Verification items for the finished model (mm, model axes). A direction names the side the tool comes from. Give positions to 0.01 mm unless a question says otherwise; leave off trailing zeros. Order: outer loops, then holes, each group sorted by start corner. A loop starts at its lowest first (then second) coordinate and runs counter-clockwise, first axis right, second up.
Autodesk Inventor part; units mm, degrees
ref_plane "YZ Plane" through (0, 0, 0) normal (1, 0, 0) x (0, 1, 0)
ref_plane "XZ Plane" through (0, 0, 0) normal (0, 1, 0) x (-1, 0, 0)
ref_plane "XY Plane" through (0, 0, 0) normal (0, 0, 1) x (1, 0, 0)
sketch "Sketch1" plane through (0, 0, 0) normal (1, 0, 0) x (0, 1, 0)
  line L0 (0, 0) -> (0, -9.15) construction
  line L1 (0, -9.15) -> (9.0687, -2.8) construction
  line L2 (9.0687, -2.8) -> (9.0687, 0) construction
  line L3 (0, -9.15) -> (0, -29.4542) construction
  line L4 (0, 0) -> (49.8191, 0) construction
  line L5 (9.0687, 0) -> (0, 0)
  line L6 (9.0687, -2.8) -> (25.35, -2.8)
  line L7 (25.35, -2.8) -> (25.35, 0)
  line L8 (25.35, 0) -> (9.0687, 0)
  line L9 (9.0687, -2.8) -> (0, -4.3991)
  line L10 (0, 0) -> (0, -4.3991)
  dimension "d1" = 125
  dimension "d2" = 5.6
  dimension "d3" = 9.15
  dimension "d5" = 9.0687
  dimension "d6" = 25.35
  dimension "d8" = 80
revolve "Revolution1" add sketch "Sketch1" angle 360 about axis through (0, 0, 0) along (0, 1, 0)
sketch "Sketch2" plane through (0, 0, 0) normal (0, -1, 0) x (1, 0, 0)
  line L0 (6.9, -13.1) -> (-16.1, -13.1) construction
  line L1 (-16.1, -13.1) -> (-16.1, 36.9)
  line L2 (-16.1, 36.9) -> (6.9, 36.9)
  line L3 (6.9, 36.9) -> (6.9, -13.1) construction
  circle A0 centre (0, 0) radius 12.5 construction
  circle A1 centre (0, 0) radius 13 construction
  line L4 (6.9, -13.1) -> (6.9, -11.0177) construction
  line L5 (6.9, 36.9) -> (6.9, 11.0177)
  line L6 (0, -13.1) -> (0, -13) construction
  line L7 (3.9, 12.4012) -> (3.9, 33.9)
  line L8 (3.9, 33.9) -> (-13.1, 33.9)
  line L9 (-13.1, 33.9) -> (-13.1, 0)
  arc A2 (6.9, 11.0177) -> (3.9, 12.4012) centre (0, 0) ccw
  arc A3 (-13.1, 0) -> (0, -13.1) centre (0, 0) ccw
  line L10 (0, -13.1) -> (0, -16.1) construction
  line L11 (-13.1, 0) -> (-13, 0) construction
  circle A4 centre (0, 0) radius 2.8
  line L12 (0, 0) -> (-13, 0) construction
  arc A5 (0, -13.1) -> (6.9, -11.0177) centre (0.1762, -1.2107) ccw
  line L13 (-13.1, 0) -> (-16.1, 0) construction
  arc A6 (-16.1, 0) -> (0, -16.1) centre (0, 0) ccw
  line L14 (6.9, -11.0177) -> (6.9, -14.0177)
  arc A7 (0, -16.1) -> (6.9, -14.0177) centre (0, -3.6267) ccw
  dimension "d9" = 25
  dimension "d10" = 0.5
  dimension "d11" = 3
  dimension "d12" = 3
  dimension "d13" = 3
  dimension "d15" = 3
  dimension "d16" = 23
  dimension "d18" = 0.1
  dimension "d19" = 0.1
  dimension "d22" = 3
  dimension "d23" = 11.8906
  dimension "d24" = 50
extrude "Extrusion1" add sketch "Sketch2" against normal up to surface (25.35 mm away) contours L1 L2 L5 A2 L7 L8 L9 A3 A5 L14 A7 A6
sketch "Sketch3" plane through (0, 0, 0) normal (0, -1, 0) x (1, 0, 0)
  line L0 (6.9, 11.0177) -> (6.9, 36.9)
  line L1 (6.9, 36.9) -> (-16.1, 36.9)
  line L2 (-16.1, 36.9) -> (-16.1, 0)
  arc A0 (-16.1, 0) -> (0, -16.1) centre (0, 0) ccw
  arc A1 (0, -16.1) -> (6.9, -14.0177) centre (0, -3.6267) ccw
  line L3 (6.9, -14.0177) -> (6.9, -11.0177)
  arc A2 (0, -13.1) -> (6.9, -11.0177) centre (0.1762, -1.2107) ccw construction
  line L4 (6.9, 11.0177) -> (6.9, -11.0177) construction
  arc A3 (6.9, -10.4177) -> (6.9, 10.4177) centre (-0.0081, 0) ccw construction
  arc A4 (6.9, -10.6569) -> (6.9, 10.6569) centre (-0.0081, 0) ccw
  line L5 (6.9, 0) -> (12.6919, 0) construction
  line L6 (6.9, -10.6569) -> (6.9, -11.0177)
  line L7 (6.9, 11.0177) -> (6.9, 10.6569)
  point P0 (0, 0)
  dimension "d29" = 12.5
  dimension "d30" = 0.2
  dimension "d31" = 0.6
extrude "Extrusion2" add sketch "Sketch3" along normal blind 3
mirror "Mirror1" about plane through (0, 25.35, 0) normal (0, 1, 0) of "Extrusion1", "Extrusion2", "Revolution1"
(1) Go/stop test with flat-tipped pins: pin 1 (21 mm diameter, centred on y = 31.5, z = 29, fed in from +X); pin 2 (1 mm diameter, centred on x = -6, y = 19.5, fed in from -Z). Record where each tip stops, or that it passes through.
Solved:
pin 1: stops at x = 6.9
pin 2: stops at z = -15.13
(2) Section check B-B, the plane y = 26.5. Enter the section's corners in (x, z), then the cut area to 3 significant figures.
Solved:
outline: (-16.1, 0) arc R16.1 ccw to (0, -16.1) arc R12.47 ccw to (6.9, -14.02) - (6.9, -11.02) arc R11.89 cw to (0, -13.1) arc R13.1 cw to (-13.1, 0) - (-13.1, 33.9) - (3.9, 33.9) - (3.9, 12.4) arc R13 cw to (6.9, 11.02) - (6.9, 36.9) - (-16.1, 36.9) - close; circle Ø5.6 at (0, 0)
area: 351 mm2
(3) Section check A-A, the plane z = 26. Enter the section's corners in (x, y).
Solved:
outline: (-16.1, -3) - (6.9, -3) - (6.9, 53.7) - (-16.1, 53.7) - close; hole (-13.1, 0) - (3.9, 0) - (3.9, 50.7) - (-13.1, 50.7) - close
(4) Set-up check for faces 1 (the flat face through (-3, 50.7, 11)), 2 (the flat face through (6.9, 25, -12)), 3 (the cylindrical face through (12.69, 52.18, -0.18)): record each of +Z, -Z, +X, -X, +Y, -Y from which the full face is reachable in a straight line by a thin tool's end or side.
Solved:
face 1: none
face 2: -Z, +X, +Y, -Y
face 3: +X, +Y, -Y
(5) Scan lines: line 1 (X direction, y = 8.5, z = 29); line 2 (Z direction, x = 2.25, y = 9); line 3 (Y direction, x = -6.75, z = 21). Record each from-to range of solid material in increasing order.
Solved:
line 1: x = -16.1 to -13.1, 3.9 to 6.9
line 2: z = -15.9 to -12.92, -1.69 to 1.69, 33.9 to 36.9
line 3: y = -3 to 0, 50.7 to 53.7
(6) Release check for a two-part mould opening along Y. For faces 4 (the flat face through (-5, 53.7, 11)), 5 (the cylindrical face through (-9.161, 25.705, -9.364)), 6 (the cylindrical face through (12.69, -1.48, 0.18)), 7 (the cylindrical face through (3.66, 25.7, -12.58)) record: pulls with the +Y half, pulls with the -Y half, needs draft (parallel to the pull), parting line crosses it, or undercut.
Solved:
face 4: pulls with the +Y half
face 5: undercut
face 6: needs draft
face 7: undercut
(7) Section check C-C, the plane x = 9. Enter the section's corners in (y, z), then the cut area to 3 significant figures.
Solved:
outline: (-3, -8.95) - (0, -8.95) - (0, 8.95) - (-3, 8.95) - close; (50.7, -8.95) - (53.7, -8.95) - (53.7, 8.95) - (50.7, 8.95) - close
area: 107 mm2
(8) Section check D-D, the plane z = 8.5. Enter the section's corners in (x, y), then the cut area to 3 significant figures.
Solved:
outline: (-16.1, -3) - (9.43, -3) - (9.43, 0) - (-13.1, 0) - (-13.1, 50.7) - (9.43, 50.7) - (9.43, 53.7) - (-16.1, 53.7) - close
area: 305 mm2
